```python
from build123d import *

# Parameters (mm, degrees)
SKETCH1_R              = 19.05
BOSS_EXTRUDE1_DEPTH    = 120
SKETCH4_R              = 11
BOSS_EXTRUDE2_DEPTH    = 10
SKETCH8_OUTSIDE_W      = 68.244
SKETCH8_OUTSIDE_H      = 68.244
SKETCH8_OUTSIDE_W_2    = 22
SKETCH8_OUTSIDE_H_2    = 38.1
CUT_EXTRUDE2_DEPTH     = 123.987011509
SKETCH2_OUTSIDE_W      = 51.448
SKETCH2_OUTSIDE_H      = 67.548
SKETCH2_OUTSIDE_W_2    = 16
SKETCH2_OUTSIDE_H_2    = 38.1
CUT_EXTRUDE1_DEPTH     = 40
M8X1_25_TAPPED_HOLE1_D = 6.8


with BuildPart() as part:
    # Sketch1 → Boss-Extrude1 (new body)
    with BuildSketch(Plane.XY):
        Circle(SKETCH1_R)
    extrude(amount=BOSS_EXTRUDE1_DEPTH)

    # Sketch4 → Boss-Extrude2 (add)
    with BuildSketch(Plane(origin=(0, 0, 0), x_dir=(-1, 0, 0), z_dir=(0, 0, -1))):
        Circle(SKETCH4_R)
    extrude(amount=BOSS_EXTRUDE2_DEPTH)

    # Sketch8 outside → Cut-Extrude2 (cut, through all)
    with BuildSketch(Plane(origin=(0, 0, 0), x_dir=(-1, 0, 0), z_dir=(0, 0, -1))):
        Rectangle(SKETCH8_OUTSIDE_W, SKETCH8_OUTSIDE_H)
        Rectangle(SKETCH8_OUTSIDE_W_2, SKETCH8_OUTSIDE_H_2, mode=Mode.SUBTRACT)
    extrude(amount=-CUT_EXTRUDE2_DEPTH, mode=Mode.SUBTRACT)

    # Sketch2 outside → Cut-Extrude1 (cut)
    with BuildSketch(Plane.XY.offset(120)):
        Rectangle(SKETCH2_OUTSIDE_W, SKETCH2_OUTSIDE_H)
        Rectangle(SKETCH2_OUTSIDE_W_2, SKETCH2_OUTSIDE_H_2, mode=Mode.SUBTRACT)
    extrude(amount=-CUT_EXTRUDE1_DEPTH, mode=Mode.SUBTRACT)

    # M8x1.25 Tapped Hole1 (through all)
    with Locations(Plane(origin=(8, 0, 0), x_dir=(0, 0, -1), z_dir=(1, 0, 0))):
        with Locations((-105, 0)):
            Hole(M8X1_25_TAPPED_HOLE1_D / 2)


solid = part.part
```
Input: part model. Units: mm. Frame: model coordinates. A direction names the side the tool comes from. Round coordinates to 2 decimals unless told otherwise and drop trailing zeros. Loops run counter-clockwise (first coordinate to the right, second up) from the corner with the lowest first, then second, coordinate; pieces in that order, holes last. Notation, with made-up numbers: M 8.5,-26 L 48.5,-26 A22 ccw 48.5,-7 Z; hole C 34.5,66.25 d9. An arc over 180 degrees is marked long. Answer in a Markdown table with one row per item. Add a question column.
1. Contact query for flat-ended pins moving along their axis: pin 1 (8 mm diameter, centred on y = -7.5, z = 88.5, fed in from -X); pin 2 (5 mm diameter, centred on x = 7.5, z = 42, fed in from -Y); pin 3 (3 mm diameter, centred on x = 8, z = 28.5, fed in from +Y). Output: stop coordinate, or through.
2. Section D-D (z = 18.5). Output: boundary loops of the cut face in (x, y), and give its area (3 significant figures).
3. Section B-B (z = 105). Output: boundary loops of the cut face in (x, y).
4. Set-up query: faces 1 (the face through (8, 0, 100)), 2 (the face through (11, 0, 39)), 3 (the face through (2.38, -10.74, -4.93)), 4 (the face through (-8, 0, 100)), 5 (the face through (0, 0, -10)). Return all of +Z, -Z, +X, -X, +Y, -Y with unobstructed straight access to the full face (end or side cutting, diameter ignored); none if empty.
5. Section A-A (x = 0). Output: boundary loops of the cut face in (y, z), and give its area (3 significant figures).
6. Section C-C (y = -12.5). Output: boundary loops of the cut face in (x, z).
7. Mould query, pull axis Z, two halves, no side actions, for faces 6 (the face through (-0.1, 0.1, 101.6)), 7 (the face through (0, 0, 120)), 8 (the face through (-11, 0, 39)), 9 (the face through (0, -14, 0)). Classes: released by +Z, released by -Z, zero draft, split by the parting line, or undercut.
8. Ray query, probe 1 along Y at (x, z) = (-1, 105); probe 2 along Y at (x, z) = (0.5, 92.5); probe 3 along Z at (x, y) = (0.25, -0.5). Return the intervals inside material, ascending.
Values follow:
| question | item | result |
|---|---|---|
| 1 | pin 1 | x = -8 |
| 1 | pin 2 | y = -18.38 |
| 1 | pin 3 | y = 17.91 |
| 2 | outline | M -11,-15.55 A19.05 ccw 11,-15.55 L 11,15.55 A19.05 ccw -11,15.55 Z |
| 2 | area | 789 mm^2 |
| 3 | outline | M -8,-17.29 A19.05 ccw 8,-17.29 L 8,-3.4 L -8,-3.4 Z; M -8,3.4 L 8,3.4 L 8,17.29 A19.05 ccw -8,17.29 Z |
| 4 | face 1 | +Z, +X, +Y, -Y |
| 4 | face 2 | +Z, -Z, +X, +Y, -Y |
| 4 | face 3 | -Z |
| 4 | face 4 | +Z, -X, +Y, -Y |
| 4 | face 5 | -Z, +X, -X, +Y, -Y |
| 5 | outline | M -19.05,0 L -11,0 L -11,-10 L 11,-10 L 11,0 L 19.05,0 L 19.05,120 L -19.05,120 Z; hole C 0,105 d6.8 |
| 5 | area | 4,760 mm^2 |
| 6 | outline | M -11,0 L 11,0 L 11,80 L 8,80 L 8,120 L -8,120 L -8,80 L -11,80 Z |
| 7 | face 6 | undercut |
| 7 | face 7 | released by +Z |
| 7 | face 8 | zero draft |
| 7 | face 9 | released by -Z |
| 8 | probe 1 | -19.02 to -3.4, 3.4 to 19.02 |
| 8 | probe 2 | -19.04 to 19.04 |
| 8 | probe 3 | -10 to 101.64, 108.36 to 120 |
